Work out the finished part from the listing and answer in its coordinate system (mm). A direction names the side the tool comes from. Round coordinates to 2 decimals unless told otherwise and drop trailing zeros. Write each loop counter-clockwise with the first axis right and the second up, starting at its lowest first coordinate (ties: lowest second). Pieces come first, ordered by that corner, then holes. Notation, with made-up numbers: (57.25, -34.5) -> (111.25, -34.5) arc R23 ccw to (111.25, -15.5) -> close; hole circle Ø8 at (-8, 13). An arc over 180 degrees is marked (long way). One line per item, written item: value.
```python
from build123d import *

# Parameters (mm, degrees)
SKETCH1_R                     = 12.9921
BOSS_EXTRUDE1_DEPTH           = 25.4
CUT_EXTRUDE1_DEPTH            = 102.12582981
CUT_EXTRUDE1_DEPTH_BACK       = 102.12582981
SKETCH3_R                     = 3.81
CUT_REVOLVE10_ANGLE           = 90
CUT_REVOLVE10_OTHER_WAY_ANGLE = 180
CUT_EXTRUDE4_DEPTH            = 32.004
FILLET1_R                     = 1.27
SKETCH15_R                    = 7.62
CUT_EXTRUDE5_DEPTH            = 10.16


with BuildPart() as part:
    # Sketch1 → Boss-Extrude1 (new body)
    with BuildSketch(Plane(origin=(0, 0, 0), x_dir=(1, 0, 0), z_dir=(0, 1, 0))):
        with Locations(Location((0, 0, 0), (0, 0, 270))):
            Circle(SKETCH1_R)
    extrude(amount=BOSS_EXTRUDE1_DEPTH)

    # Sketch2 → Revolve1 (revolve)
    with BuildSketch(Plane(origin=(0, 0, 0), x_dir=(0, 0, -1), z_dir=(1, 0, 0))):
        with BuildLine():
            Line((-16.764, 25.4), (-16.764, 49.53))
            ThreePointArc((-16.764, 49.53), (-11.85393808, 61.38393808), (0, 66.294))
            Line((0, 66.294), (0, 25.4))
            Line((0, 25.4), (-16.764, 25.4))
        make_face()
    revolve(axis=Axis((0, 25.4, 0), (0, 1, 0)))

    # Sketch3 → Cut-Extrude1 (cut, two sides: drawn at the far end of the back side and taken through both)
    with BuildSketch(Plane(origin=(0, 98.307528007, 0), x_dir=(0, 0, -1), z_dir=(-1, 0, 0)).offset(-CUT_EXTRUDE1_DEPTH_BACK)):
        with Locations(Location((0, 48.777528007, 0), (0, 0, 180))):
            Circle(SKETCH3_R)
    extrude(amount=CUT_EXTRUDE1_DEPTH + CUT_EXTRUDE1_DEPTH_BACK, mode=Mode.SUBTRACT)

    # Sketch11 → Cut-Revolve10 (revolve, cut)
    with BuildSketch(Plane.XY):
        with BuildLine():
            Line((-7.62, 49.53), (-7.62, 66.294481054))
            ThreePointArc((-7.62, 66.294481054), (0, 67.945), (7.62, 66.294481054))
            Line((7.62, 66.294481054), (7.62, 49.53))
            Line((7.62, 49.53), (-7.62, 49.53))
        make_face()
    revolve(axis=Axis((16.764, 49.53, 0), (-1, 0, 0)), revolution_arc=CUT_REVOLVE10_ANGLE, mode=Mode.SUBTRACT)

    # Sketch11 → Cut-Revolve10 other way (revolve, cut)
    with BuildSketch(Plane.XY):
        with BuildLine():
            Line((-7.62, 49.53), (-7.62, 66.294481054))
            ThreePointArc((-7.62, 66.294481054), (0, 67.945), (7.62, 66.294481054))
            Line((7.62, 66.294481054), (7.62, 49.53))
            Line((7.62, 49.53), (-7.62, 49.53))
        make_face()
    revolve(axis=Axis((16.764, 49.53, 0), (1, 0, 0)), revolution_arc=CUT_REVOLVE10_OTHER_WAY_ANGLE, mode=Mode.SUBTRACT)

    # Sketch13 → Cut-Revolve11 (revolve, cut)
    with BuildSketch(Plane.XY):
        with BuildLine():
            Line((-7.62, 53.34), (7.62, 53.34))
            Line((7.62, 53.34), (7.62, 70.104481054))
            ThreePointArc((7.62, 70.104481054), (0, 71.755), (-7.62, 70.104481054))
            Line((-7.62, 70.104481054), (-7.62, 53.34))
        make_face()
    revolve(axis=Axis((-7.62, 53.34, 0), (1, 0, 0)), mode=Mode.SUBTRACT)

    # Sketch14 → Cut-Extrude4 (cut)
    with BuildSketch(Plane.XY):
        with BuildLine():
            Line((-7.62, 49.53), (-7.62, 42.063955264))
            ThreePointArc((-7.62, 42.063955264), (0, 38.862), (7.62, 42.063955264))
            Line((7.62, 42.063955264), (7.62, 49.53))
            Line((7.62, 49.53), (-7.62, 49.53))
        make_face()
    extrude(amount=-CUT_EXTRUDE4_DEPTH, mode=Mode.SUBTRACT)

    # Fillet1
    fillet1_edges = [part.edges().sort_by_distance(p)[0] for p in [
        (7.62, 35.232956393, 8.754562759),
        (-7.62, 35.232956393, 8.754562759),
        (-7.62, 38.008906377, -6.782727573),
        (7.62, 38.008906377, -6.782727573),
        (-7.62, 42.063955264, -13.66883927),
        (7.62, 42.063955264, -13.66883927),
    ]]
    fillet(fillet1_edges, radius=FILLET1_R)

    # Sketch15 → Cut-Extrude5 (cut)
    with BuildSketch(Plane(origin=(-15.24, 0, 0), x_dir=(0, 0, -1), z_dir=(-1, 0, 0))):
        with Locations((0, -49.53)):
            Circle(SKETCH15_R)
    cut_extrude5 = extrude(amount=CUT_EXTRUDE5_DEPTH, mode=Mode.SUBTRACT)

    # Mirror1: Cut-Extrude5 across plane
    add(cut_extrude5.mirror(Plane.ZY), mode=Mode.SUBTRACT)


solid = part.part
```
(1) Flat-ended cylindrical pins translate along their axes: pin 1 Ø1 at (x, z) = (-10, 12) entering from +Y; pin 2 Ø1 at (x, z) = (-0.5, -7) entering from -Y; pin 3 Ø1 at (x, y) = (2.5, 26) entering from -Z; pin 4 Ø4.5 at (y, z) = (49.53, 0) entering from +X. Find the tip coordinate at first contact, or state that the pin passes through.
Reported:
pin 1: stops at y = 56.77
pin 2: stops at y = 0
pin 3: stops at z = -16.64
pin 4: passes through
(2) Consider probe 1 along X at (y, z) = (51.5, 3.5); probe 2 along Y at (x, z) = (-11, 0); probe 3 along X at (y, z) = (59.5, -3.5). Determine where each line is inside the solid, lowest interval first.
Reported:
probe 1: x = -15.24 to -7.62, 7.62 to 15.24
probe 2: y = 0 to 45.72, 53.34 to 62.18
probe 3: x = -13.01 to -7.62, 7.62 to 13.01
(3) Find section D-D on z = 2.5. Give the number of separate pieces and of enclosed holes in the cut face, plus the area to 3 significant figures.
Reported:
separate pieces: 3
enclosed holes: 0
area: 1,250 mm2
(4) Find section C-C on x = 0. Give the vertices of the cut face in (y, z) (3 decimals).
Reported:
outline: (0, -12.992) -> (25.4, -12.992) -> (25.4, -16.764) -> (38.862, -16.764) -> (38.862, -11.38) arc R18.415 cw to (34.925, 0) -> (31.115, 0) arc R18.415 cw to (41.909, 16.764) -> (25.4, 16.764) -> (25.4, 12.992) -> (0, 12.992) -> close
(5) Find section B-B on y = 55.5. Give the vertices of the cut face in (x, z), plus the area to 3 significant figures.
Reported:
outline: (-15.24, -3.62) arc R15.66 ccw to (-7.62, -13.69) -> (-7.62, 13.69) arc R15.66 ccw to (-15.24, 3.62) -> close; (7.62, -13.69) arc R15.66 ccw to (15.24, -3.62) -> (15.24, 3.62) arc R15.66 ccw to (7.62, 13.69) -> close
area: 309 mm2
(6) Find section A-A on x = 10. Give the vertices of the cut face in (y, z).
Reported:
outline: (0, -8.29) -> (25.4, -8.29) -> (25.4, -13.45) -> (49.53, -13.45) arc R13.45 ccw to (49.53, 13.45) -> (25.4, 13.45) -> (25.4, 8.29) -> (0, 8.29) -> close; hole circle Ø7.62 at (49.53, 0)
(7) A tool of negligible diameter and unlimited length cuts with its end or side. For faces 4 (the face through (11.48, 45.81, -0.83)), 5 (the face through (-15.82, 41.91, -0.12)), 6 (the face through (-7.62, 53, 4)), 7 (the face through (-0.111, 38.863, -14.035)), 8 (the face through (15.24, 46, 2)), from which of +Z, -Z, +X, -X, +Y, -Y can it reach the whole face along a straight path? Write none if from no direction.
Reported:
face 4: +X, -X
face 5: -X, +Y
face 6: +Y
face 7: -Z, +Y
face 8: +X, +Y
(8) For a pull along Z with two mould halves and no side action, classify faces 1 (the face through (-15.24, 46, 2)), 2 (the face through (3.902, 12.522, 12.392)), 3 (the face through (-10, 25.4, -9)) as pulls with the +Z half, pulls with the -Z half, needs draft (parallel to the pull), parting line crosses it, or undercut.
Reported:
face 1: undercut
face 2: parting line crosses it
face 3: needs draft
